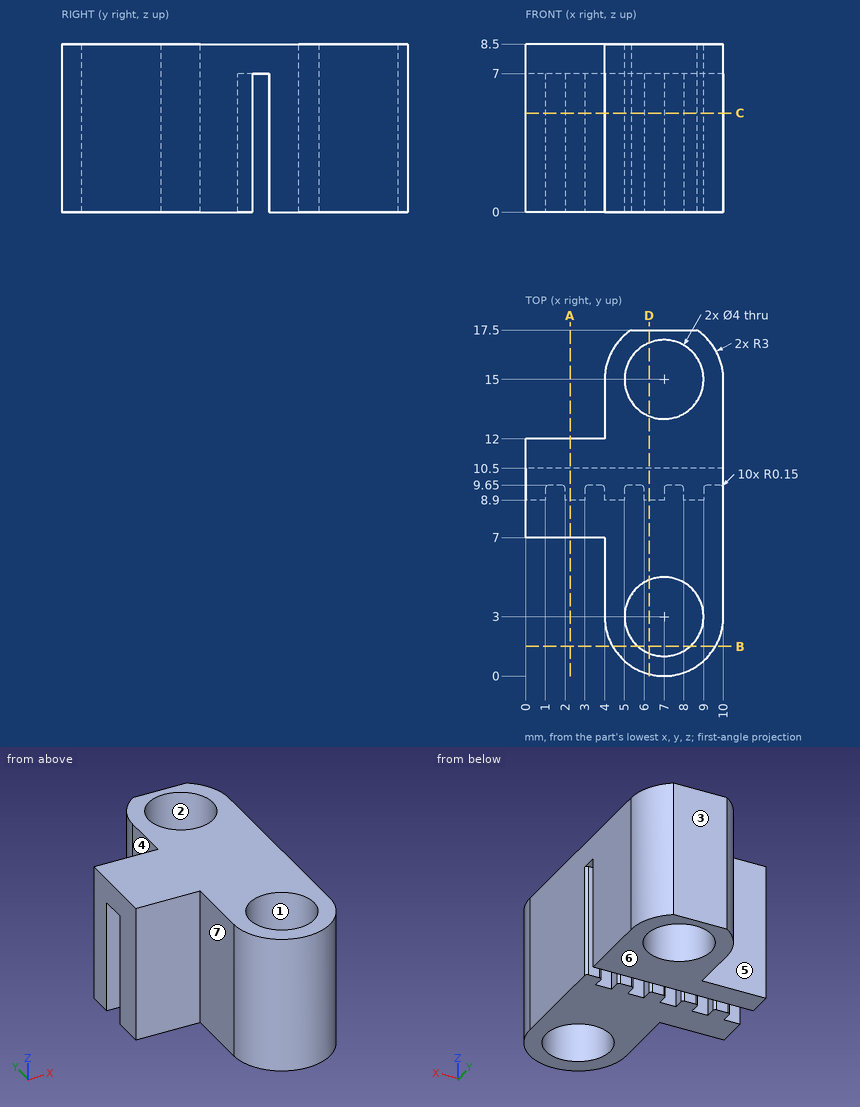
Answer from the drawing. Dimensions are ordinates in mm from the lowest x, y and z of the part. A direction names the side the tool comes from. Round coordinates to 2 decimals unless told otherwise and drop trailing zeros. Loops run counter-clockwise (first coordinate to the right, second up) from the corner with the lowest first, then second, coordinate; pieces in that order, holes last.
(1) Find the intervals of material crossed by L1, parallel to Y at x = 7, z = 8; L2, parallel to Y at x = 5.25, z = 1.25; L3, parallel to Y at x = 3.5, z = 4.75, in increasing order.
Computed values:
L1: y = 0 to 1, 5 to 13, 17 to 17.5
L2: y = 0.56 to 2.03, 3.97 to 9.65, 10.5 to 14.03, 15.97 to 17.44
L3: y = 7 to 9.65, 10.5 to 12
(2) Each of these flat-tipped pins is pushed along its axis until it touches: P1, Ø1.2, axis at y = 5, z = 5, coming from the -X side; P2, Ø2, axis at x = 2.5, z = 5.5, coming from the +Y side; P3, Ø0.5, axis at y = 9.5, z = 4, coming from the -X side. Where does it stop, or does it pass through?
Computed values:
P1: stops at x = 4
P2: stops at y = 12
P3: stops at x = 1
(3) The part is cut by section A-A, the plane x = 2.25. Give the vertices of the cut face in (y, z).
Computed values:
outline: (7, 0) - (8.9, 0) - (8.9, 7) - (10.5, 7) - (10.5, 0) - (12, 0) - (12, 8.5) - (7, 8.5) - close
(4) The part is cut by section B-B, the plane y = 1.5. Give the vertices of the cut face in (x, z).
Computed values:
outline: (4.4, 0) - (5.68, 0) - (5.68, 8.5) - (4.4, 8.5) - close; (8.32, 0) - (9.6, 0) - (9.6, 8.5) - (8.32, 8.5) - close
(5) The mould has two halves that part along Y. Classify the marked faces 1, 2, 3 and 4: pulls with the +Y half, pulls with the -Y half, needs draft (parallel to the pull), parting line crosses it, or undercut.
Computed values:
face 1: undercut
face 2: undercut
face 3: pulls with the +Y half
face 4: needs draft
(6) The part is cut by section D-D, the plane x = 6.25. Give the vertices of the cut face in (y, z).
Computed values:
outline: (0.1, 0) - (1.15, 0) - (1.15, 8.5) - (0.1, 8.5) - close; (4.85, 0) - (8.9, 0) - (8.9, 7) - (10.5, 7) - (10.5, 0) - (13.15, 0) - (13.15, 8.5) - (4.85, 8.5) - close; (16.85, 0) - (17.5, 0) - (17.5, 8.5) - (16.85, 8.5) - close
(7) The part is cut by section C-C, the plane z = 5. Give the number of separate pieces and of enclosed holes in the cut face, and give its area (3 significant figures).
Computed values:
separate pieces: 2
enclosed holes: 2
area: 81.7 mm2
(8) For the marked faces 5, 6 and 7, determine the directions among +Z, -Z, +X, -X, +Y, -Y from which every point of the face is accessible in a straight line to the end or side of a thin tool.
Computed values:
face 5: +Z, -Z, -X, +Y
face 6: -Z, +X, -X, +Y, -Y
face 7: +Z, -Z, -X, -Y
